Geometry: final body of the model. Coordinates: model frame, mm. Face numbers are marked on the shaded views. A direction names the side the tool comes from. Give positions to 0.01 mm unless a question says otherwise; leave off trailing zeros. Write each loop counter-clockwise with the first axis right and the second up, starting at its lowest first coordinate (ties: lowest second). Pieces come first, ordered by that corner, then holes. Notation, with made-up numbers: (18, 84) -> (38, 84) arc R26 ccw to (38, 100) -> close; hole circle Ø8 at (78, 36.25). An arc over 180 degrees is marked (long way). Answer in a Markdown table with one row per item. Add a question column.
Item 1: Material intervals for probe 1 along Y at (x, z) = (7, 0); probe 2 along X at (y, z) = (-1.6, -2); probe 3 along Z at (x, y) = (7, -0.7), sorted ascending. Write a range as from..to.
Item 2: Access query for the marked faces 4 and 5. Directions: +Z, -Z, +X, -X, +Y, -Y. A direction counts if a zero-diameter tool reaches every point of the face in a straight line with its end or side. Return the directions, or none.
Item 3: Draft query along Z for the marked faces 1, 2 and 3. Return one class per face: +Z half, -Z half, draft (parallel to the pull), parting line (faces both ways), or undercut.
Item 4: Section query D-D on z = 0.5. Output: boundary loops of the cut face in (x, y).
Item 5: Section query A-A on x = 6.5. Output: boundary loops of the cut face in (y, z), plus the area to 3 significant figures.
Item 6: Section query C-C on x = -4.5. Output: boundary loops of the cut face in (y, z).
Item 7: Section query B-B on y = -0.7. Output: boundary loops of the cut face in (x, z).
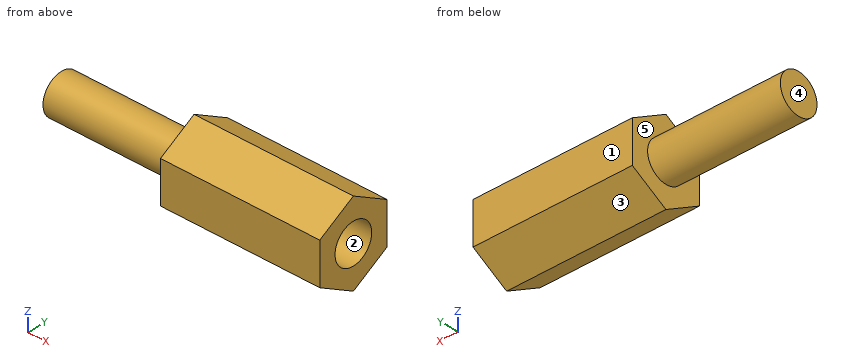
```python
from build123d import *

# Parameters (mm, degrees)
SKETCH2_R                = 1.5
BOSS_EXTRUDE1_DEPTH      = 12
BOSS_EXTRUDE2_DEPTH      = 10
BOSS_EXTRUDE2_DEPTH_BACK = 2
SKETCH3_R                = 1.5


with BuildPart() as part:
    # Sketch2 → Boss-Extrude1 (new body)
    with BuildSketch(Plane(origin=(0, 0, 0), x_dir=(0, 0, -1), z_dir=(1, 0, 0))):
        Polygon((1.58771324, 2.75), (-1.58771324, 2.75), (-3.175426481, 0), (-1.58771324, -2.75), (1.58771324, -2.75), (3.175426481, 0), align=None)
        Circle(SKETCH2_R, mode=Mode.SUBTRACT)
    extrude(amount=BOSS_EXTRUDE1_DEPTH)

    # Sketch3 → Boss-Extrude2 (add, two sides: drawn at the far end of the back side and taken through both)
    with BuildSketch(Plane.ZY.offset(-BOSS_EXTRUDE2_DEPTH_BACK)):
        Circle(SKETCH3_R)
    extrude(amount=BOSS_EXTRUDE2_DEPTH + BOSS_EXTRUDE2_DEPTH_BACK)


solid = part.part
```
Findings below:
| question | item | result |
|---|---|---|
| 1 | probe 1 | y = -2.75..-1.5, 1.5..2.75 |
| 1 | probe 2 | x = 0..12 |
| 1 | probe 3 | z = -2.77..-1.33, 1.33..2.77 |
| 2 | face 4 | +Z, -Z, -X, +Y, -Y |
| 2 | face 5 | -X |
| 3 | face 1 | draft |
| 3 | face 2 | undercut |
| 3 | face 3 | -Z half |
| 4 | outline | (-10, -1.41) -> (0, -1.41) -> (0, -2.75) -> (12, -2.75) -> (12, -1.41) -> (2, -1.41) -> (2, 1.41) -> (12, 1.41) -> (12, 2.75) -> (0, 2.75) -> (0, 1.41) -> (-10, 1.41) -> close |
| 5 | outline | (-2.75, -1.59) -> (0, -3.18) -> (2.75, -1.59) -> (2.75, 1.59) -> (0, 3.18) -> (-2.75, 1.59) -> close; hole circle Ø3 at (0, 0) |
| 5 | area | 19.1 mm^2 |
| 6 | outline | circle Ø3 at (0, 0) |
| 7 | outline | (-10, -1.33) -> (0, -1.33) -> (0, -2.77) -> (12, -2.77) -> (12, -1.33) -> (2, -1.33) -> (2, 1.33) -> (12, 1.33) -> (12, 2.77) -> (0, 2.77) -> (0, 1.33) -> (-10, 1.33) -> close |
